from build123d import *

# Parameters (mm, degrees)
SKETCH1_R           = 2.1
BOSS_EXTRUDE1_DEPTH = 1.2
FILLET1_R           = 5


with BuildPart() as part:
    # Sketch1 → Boss-Extrude1 (new body)
    with BuildSketch(Plane.XY):
        Polygon((-56.4, 136.5), (-56.4, 114.638335016), (56.4, 114.638335016), (56.4, 136.5), (0, 136.5), align=None)
        with Locations((0, 127)):
            Circle(SKETCH1_R, mode=Mode.SUBTRACT)
    extrude(amount=BOSS_EXTRUDE1_DEPTH)

    # Fillet1
    fillet1_edges = [part.edges().sort_by_distance(p)[0] for p in [
        (56.4, 114.638335016, 0.6),
        (-56.4, 114.638335016, 0.6),
        (-56.4, 136.5, 0.6),
        (56.4, 136.5, 0.6),
    ]]
    fillet(fillet1_edges, radius=FILLET1_R)


solid = part.part
Geometry: final body of the model. Coordinates: model frame, mm. Round coordinates to 2 decimals unless told otherwise and drop trailing zeros. Order: outer loops, then holes, each group sorted by start corner. A loop starts at its lowest first (then second) coordinate and runs counter-clockwise, first axis right, second up.
Q1. Material intervals for probe 1 along Y at (x, z) = (0, 0.6); probe 2 along X at (y, z) = (125.5, 0.7); probe 3 along X at (y, z) = (127.5, 0.4), sorted ascending.
Result sheet:
probe 1: y = 114.64 to 124.9, 129.1 to 136.5
probe 2: x = -56.4 to -1.47, 1.47 to 56.4
probe 3: x = -56.4 to -2.04, 2.04 to 56.4
Q2. Section A-A, the plane x = 0. Output: boundary loops of the cut face in (y, z), and give its area (3 significant figures).
Result sheet:
outline: (114.64, 0) - (124.9, 0) - (124.9, 1.2) - (114.64, 1.2) - close; (129.1, 0) - (136.5, 0) - (136.5, 1.2) - (129.1, 1.2) - close
area: 21.2 mm2
Q3. Mould query, pull axis X, two halves, no side actions, for faces 1 (the face through (-54.97, 135, 0.61)), 2 (the face through (54.896, 116.064, 0.608)), 3 (the face through (-1, 123, 0)), 4 (the face through (-0.46, 124.95, 0.59)). Classes: released by +X, released by -X, zero draft, split by the parting line, or undercut.
Result sheet:
face 1: released by -X
face 2: released by +X
face 3: zero draft
face 4: undercut
Q4. Section B-B, the plane y = 127. Output: boundary loops of the cut face in (x, z), and give its area (3 significant figures).
Result sheet:
outline: (-56.4, 0) - (-2.1, 0) - (-2.1, 1.2) - (-56.4, 1.2) - close; (2.1, 0) - (56.4, 0) - (56.4, 1.2) - (2.1, 1.2) - close
area: 130 mm2
